Autodesk Inventor part; units mm, degrees
ref_plane "YZ Plane" through (0, 0, 0) normal (1, 0, 0) x (0, 1, 0)
ref_plane "XZ Plane" through (0, 0, 0) normal (0, 1, 0) x (-1, 0, 0)
ref_plane "XY Plane" through (0, 0, 0) normal (0, 0, 1) x (1, 0, 0)
sketch "Sketch1" plane through (0, 0, 0) normal (0, 1, 0) x (-1, 0, 0)
  circle A0 centre (0, 0) radius 11.125
  circle A1 centre (0, 0) radius 13.125
  dimension "d0" = 22.25
  dimension "d1" = 26.25
extrude "Extrusion1" add sketch "Sketch1" along normal blind 60
sketch "Sketch2" plane through (0, 60, 0) normal (0, 1, 0) x (1, 0, 0)
  circle A0 centre (0, 0) radius 11.125
extrude "Extrusion2" add sketch "Sketch2" against normal blind 53
sketch "Sketch3" plane through (0, 60, 0) normal (0, 1, 0) x (1, 0, 0)
  circle A0 centre (0, 0) radius 11.125
extrude "Extrusion3" cut sketch "Sketch3" against normal blind 7
properties part number "Fretter"
Input: part model. Units: mm. Frame: model coordinates. A direction names the side the tool comes from. Coordinates: 2 decimals unless noted, no trailing zeros. Loops run counter-clockwise (first coordinate to the right, second up) from the corner with the lowest first, then second, coordinate; pieces in that order, holes last. Notation, with made-up numbers: (9.25, 26.25) -> (32.25, 26.25) arc R19 cw to (32.25, 60.25) -> close; hole circle Ø11 at (37.25, -16.75). An arc over 180 degrees is marked (long way). Use a Markdown table: item, result.
1) Cut plane C-C (y = 12). Return the cut outline in (x, z) (3 decimals).
Results found:
| item | result |
|---|---|
| outline | circle Ø26.25 at (0, 0) |
2) Cut plane A-A (x = 0). Return the cut outline in (y, z) (3 decimals).
Results found:
| item | result |
|---|---|
| outline | (0, -13.125) -> (60, -13.125) -> (60, -11.125) -> (53, -11.125) -> (53, 11.125) -> (60, 11.125) -> (60, 13.125) -> (0, 13.125) -> (0, 11.125) -> (7, 11.125) -> (7, -11.125) -> (0, -11.125) -> close |
3) Access query for faces 1 (the flat face through (11, 60, 3)), 2 (the flat face through (0, 53, 0)), 3 (the flat face through (0, 7, 0)). Directions: +Z, -Z, +X, -X, +Y, -Y. A direction counts if a zero-diameter tool reaches every point of the face in a straight line with its end or side. Return the directions, or none.
Results found:
| item | result |
|---|---|
| face 1 | +Z, -Z, +X, -X, +Y |
| face 2 | +Y |
| face 3 | -Y |
4) Cut plane B-B (z = 0). Return the cut outline in (x, y) (3 decimals), then the cut area to 3 significant figures.
Results found:
| item | result |
|---|---|
| outline | (-13.125, 0) -> (-11.125, 0) -> (-11.125, 7) -> (11.125, 7) -> (11.125, 0) -> (13.125, 0) -> (13.125, 60) -> (11.125, 60) -> (11.125, 53) -> (-11.125, 53) -> (-11.125, 60) -> (-13.125, 60) -> close |
| area | 1,260 mm2 |
5) Pull-direction query (Z, two-part tool) for faces 4 (the cylindrical face through (-8.2, 56.55, -7.52)), 5 (the flat face through (11, 0, 3)), 6 (the cylindrical face through (-12.52, 29.58, -3.94)); classes: released by +Z, released by -Z, zero draft, split by the parting line, or undercut.
Results found:
| item | result |
|---|---|
| face 4 | undercut |
| face 5 | zero draft |
| face 6 | split by the parting line |
6) Contact query for flat-ended pins moving along their axis: pin 1 (2 mm diameter, centred on x = -8, y = 51.5, fed in from -Z); pin 2 (3 mm diameter, centred on y = 48.5, z = -3.5, fed in from +X); pin 3 (3 mm diameter, centred on y = 32, z = -2.5, fed in from -X). Output: stop coordinate, or through.
Results found:
| item | result |
|---|---|
| pin 1 | stops at z = -11.1 |
| pin 2 | stops at x = 12.97 |
| pin 3 | stops at x = -13.09 |
7) Material intervals for line 1 along Z through (x, y) = (0, 3.25) (3 decimals); line 2 along Y through (x, z) = (-6.25, -0.5); line 3 along X through (y, z) = (19.5, -3), sorted ascending. Write a range as from..to.
Results found:
| item | result |
|---|---|
| line 1 | z = -13.125..-11.125, 11.125..13.125 |
| line 2 | y = 7..53 |
| line 3 | x = -12.78..12.78 |
